```python
from build123d import *

# Parameters (mm, degrees)
SKETCH_1_W          = 70
SKETCH_1_H          = 25
EXTRUDE_1_DEPTH     = 4
SKETCH_2_W          = 5
SKETCH_2_H          = 25
EXTRUDE_2_DEPTH     = 20
SKETCH_3_W          = 70
SKETCH_3_H          = 25
EXTRUDE_3_DEPTH     = 4
SKETCH_4_R          = 1.6
CUT_EXTRUDE_1_DEPTH = 4
SKETCH_5_R          = 3.5
CUT_EXTRUDE_2_DEPTH = 3
SKETCH_6_R          = 3.5
CUT_EXTRUDE_3_DEPTH = 45.240818256
CUT_EXTRUDE_4_DEPTH = 47.532246883
FILLET_1_R          = 10
SKETCH_8_R          = 2.25
CUT_EXTRUDE_5_DEPTH = 77.42152838
FILLET_2_R          = 1
FILLET_3_R          = 5


with BuildPart() as part:
    # Эскиз1 → Бобышка-Вытянуть1 (new body)
    with BuildSketch(Plane(origin=(0, 0, 0), x_dir=(1, 0, 0), z_dir=(0, 1, 0))):
        Rectangle(SKETCH_1_W, SKETCH_1_H)
    extrude(amount=EXTRUDE_1_DEPTH)

    # Эскиз2 → Бобышка-Вытянуть2 (add)
    with BuildSketch(Plane(origin=(0, 4, 0), x_dir=(1, 0, 0), z_dir=(0, 1, 0))):
        with Locations((32.5, 0)):
            Rectangle(SKETCH_2_W, SKETCH_2_H)
    extrude(amount=EXTRUDE_2_DEPTH)

    # Эскиз3 → Бобышка-Вытянуть3 (add)
    with BuildSketch(Plane(origin=(0, 24, 0), x_dir=(1, 0, 0), z_dir=(0, 1, 0))):
        Rectangle(SKETCH_3_W, SKETCH_3_H)
    extrude(amount=EXTRUDE_3_DEPTH)

    # Эскиз4 → Вырез-Вытянуть1 (cut)
    with BuildSketch(Plane.XZ):
        with Locations(Location((5, 0, 0), (0, 0, 270))):
            Circle(SKETCH_4_R)
    extrude(amount=-CUT_EXTRUDE_1_DEPTH, mode=Mode.SUBTRACT)

    # Эскиз5 → Вырез-Вытянуть2 (cut)
    with BuildSketch(Plane(origin=(0, 4, 0), x_dir=(1, 0, 0), z_dir=(0, 1, 0))):
        with Locations(Location((5, 0, 0), (0, 0, 270))):
            Circle(SKETCH_5_R)
    extrude(amount=-CUT_EXTRUDE_2_DEPTH, mode=Mode.SUBTRACT)

    # Эскиз6 → Вырез-Вытянуть3 (cut, through all)
    with BuildSketch(Plane.XZ.offset(-24)):
        with Locations(Location((5, 0, 0), (0, 0, 90))):
            Circle(SKETCH_6_R)
    extrude(amount=-CUT_EXTRUDE_3_DEPTH, mode=Mode.SUBTRACT)

    # Эскиз7 → Вырез-Вытянуть4 (cut, through all)
    with BuildSketch(Plane(origin=(0, 28, 0), x_dir=(1, 0, 0), z_dir=(0, 1, 0))):
        with BuildLine():
            Line((-31, 1.5), (-1, 1.5))
            ThreePointArc((-1, 1.5), (0.5, 0), (-1, -1.5))
            Line((-1, -1.5), (-31, -1.5))
            ThreePointArc((-31, -1.5), (-32.5, 0), (-31, 1.5))
        make_face()
    extrude(amount=-CUT_EXTRUDE_4_DEPTH, mode=Mode.SUBTRACT)

    # Скругление1
    fillet_1_edges = [part.edges().sort_by_distance(p)[0] for p in [
        (-35, 26, -12.5),
        (-35, 26, 12.5),
        (-35, 2, 12.5),
        (-35, 2, -12.5),
    ]]
    fillet(fillet_1_edges, radius=FILLET_1_R)

    # Эскиз8 → Вырез-Вытянуть5 (cut, through all)
    with BuildSketch(Plane(origin=(35, 0, 0), x_dir=(0, 0, -1), z_dir=(1, 0, 0))):
        with Locations((0, 14)):
            Circle(SKETCH_8_R)
    extrude(amount=-CUT_EXTRUDE_5_DEPTH, mode=Mode.SUBTRACT)

    # Скругление2
    fillet_2_edges = [part.edges().sort_by_distance(p)[0] for p in [
        (30, 4, 0),
        (30, 24, 0),
    ]]
    fillet(fillet_2_edges, radius=FILLET_2_R)

    # Скругление3
    fillet_3_edges = [part.edges().sort_by_distance(p)[0] for p in [
        (35, 28, 0),
        (35, 0, 0),
    ]]
    fillet(fillet_3_edges, radius=FILLET_3_R)


solid = part.part
```
The listing builds one solid part. Answer for the finished solid, in the listing's coordinates (mm). A direction names the side the tool comes from. Give positions to 0.01 mm unless a question says otherwise; leave off trailing zeros. Order: outer loops, then holes, each group sorted by start corner. A loop starts at its lowest first (then second) coordinate and runs counter-clockwise, first axis right, second up. Notation, with made-up numbers: M 33,14 L 77,14 A21 cw 77,52 Z; hole C -36.75,79 d5. An arc over 180 degrees is marked long. Put each result on its own line as item: value. Start each with the question number.
Item 1: The part is cut by section A-A, the plane y = 14. Determine the outline of the cut face in (x, z).
Item 2: The part is cut by section B-B, the plane x = -20. Determine the outline of the cut face in (y, z).
Item 3: The part is cut by section D-D, the plane z = -5. Determine the outline of the cut face in (x, y), and give its area (3 significant figures).
Item 4: Which of the six approach directions +Z, -Z, +X, -X, +Y, -Y give full straight-line access (tool end or side, diameter ignored) to faces 4 (the face through (-35, 2, 0)), 5 (the face through (0.5, 26, 0))?
Item 5: Find the intervals of material crossed by line 1 along Y through (x, z) = (20.5, -4); line 2 along X through (y, z) = (3, -1); line 3 along X through (y, z) = (25, 0), in increasing order.
Item 6: Flat-ended cylindrical pins translate along their axes: P1, Ø5.5, axis at x = 5, z = 0, coming from the +Y side; P2, Ø6, axis at y = 14, z = 0, coming from the -X side; P3, Ø3, axis at x = 5, z = 0, coming from the -Y side. Find the tip coordinate at first contact, or state that the pin passes through.
Item 7: The part is cut by section C-C, the plane z = 0. State how many separate pieces and enclosed holes the cut face has, and give its area (3 significant figures).
Item 8: For a pull along Z with two mould halves and no side action, classify faces 1 (the face through (0.5, 2, 0)), 2 (the face through (-31.99, 2.03, -9.65)), 3 (the face through (9.3, 24.3, 12.5)) as +Z half, -Z half, draft (parallel to the pull), parting line (faces both ways), or undercut.
Answer key:
1. outline: M 30,-12.5 L 35,-12.5 L 35,-2.25 L 30,-2.25 Z; M 30,2.25 L 35,2.25 L 35,12.5 L 30,12.5 Z
2. outline: M 0,-12.5 L 4,-12.5 L 4,-1.5 L 0,-1.5 Z; M 0,1.5 L 4,1.5 L 4,12.5 L 0,12.5 Z; M 24,-12.5 L 28,-12.5 L 28,-1.5 L 24,-1.5 Z; M 24,1.5 L 28,1.5 L 28,12.5 L 24,12.5 Z
3. outline: M -34.68,0 L 30,0 A5 ccw 35,5 L 35,23 A5 ccw 30,28 L -34.68,28 L -34.68,24 L 29,24 A1 cw 30,23 L 30,5 A1 cw 29,4 L -34.68,4 Z
3. area: 647 mm²
4. face 4: +Z, -Z, -X, +Y, -Y
4. face 5: +Y, -Y
5. line 1: y = 0 to 4, 24 to 28
5. line 2: x = -35 to -32.12, 0.12 to 1.65, 8.35 to 34.58
5. line 3: x = -35 to -32.5, 0.5 to 1.5, 8.5 to 34.58
6. P1: stops at y = 1
6. P2: stops at x = 30
6. P3: passes through
7. separate pieces: 6
7. enclosed holes: 0
7. area: 311 mm²
8. face 1: undercut
8. face 2: -Z half
8. face 3: +Z half
